```python
from build123d import *

# Parameters (mm, degrees)
RING_BASE_PROFILE_R        = 80.875
RING_BASE_PROFILE_R_2      = 70.375
RING_BASE_EXTRUSTION_DEPTH = 1.5
RING_LIP_PROFILE_W         = 0.8
RING_LIP_PROFILE_H         = 4
LED_CHANNEL_PROFILE_R      = 79.425
LED_CHANNEL_PROFILE_R_2    = 71.825
LED_CHANNEL_CUT_DEPTH      = 0.75


with BuildPart() as part:
    # Ring Base Profile → Ring Base Extrustion (new body)
    with BuildSketch(Plane(origin=(0, 0, 0), x_dir=(1, 0, 0), z_dir=(0, 1, 0))):
        with Locations(Location((0, 0, 0), (0, 0, 270))):
            Circle(RING_BASE_PROFILE_R)
        with Locations(Location((0, 0, 0), (0, 0, 270))):
            Circle(RING_BASE_PROFILE_R_2, mode=Mode.SUBTRACT)
    extrude(amount=RING_BASE_EXTRUSTION_DEPTH)

    # Ring Lip: sweep along a curve in space
    with BuildLine() as ring_lip_path:
        ThreePointArc((0, 1.5, 80.875), (57.187260928, 1.5, 57.187260928), (80.875, 1.5, 0))
        ThreePointArc((80.875, 1.5, 0), (57.187260928, 1.5, -57.187260928), (0, 1.5, -80.875))
        ThreePointArc((0, 1.5, -80.875), (-57.187260928, 1.5, -57.187260928), (-80.875, 1.5, 0))
        ThreePointArc((-80.875, 1.5, 0), (-57.187260928, 1.5, 57.187260928), (0, 1.5, 80.875))
    # Ring Lip Profile → Ring Lip (sweep)
    with BuildSketch(Plane.XY):
        with BuildLine():
            Line((-80.875, 1.5), (-80.875, -0.35))
            ThreePointArc((-80.875, -0.35), (-81.275, -0.75), (-80.875, -1.15))
            Line((-80.875, -1.15), (-80.875, -2.5))
            Line((-80.875, -2.5), (-81.675, -2.5))
            Line((-81.675, -2.5), (-81.675, 1.5))
            Line((-81.675, 1.5), (-80.875, 1.5))
        make_face()
        with Locations((-69.975, -0.5)):
            Rectangle(RING_LIP_PROFILE_W, RING_LIP_PROFILE_H)
    sweep(path=ring_lip_path.line)

    # LED Channel Profile → LED Channel Cut (cut)
    with BuildSketch(Plane.XZ):
        with Locations(Location((0, 0, 0), (0, 0, 270))):
            Circle(LED_CHANNEL_PROFILE_R)
        with Locations(Location((0, 0, 0), (0, 0, 270))):
            Circle(LED_CHANNEL_PROFILE_R_2, mode=Mode.SUBTRACT)
    extrude(amount=-LED_CHANNEL_CUT_DEPTH, mode=Mode.SUBTRACT)


solid = part.part
```
Design review of the part built by this model. Coordinates are the model's own, in mm. A direction names the side the tool comes from. Round coordinates to 2 decimals unless told otherwise and drop trailing zeros. Write each loop counter-clockwise with the first axis right and the second up, starting at its lowest first coordinate (ties: lowest second). Pieces come first, ordered by that corner, then holes. Notation, with made-up numbers: (71.5, 43.25) -> (107.5, 43.25) arc R19 cw to (107.5, 68.25) -> close; hole circle Ø9 at (65, 87.25). An arc over 180 degrees is marked (long way). Write item = value, one per line. Start each with the question number.
1) Mouldability with a two-part tool opening along Z and no side actions: class faces 3 (the face through (-53, 0, 48)), 4 (the face through (-59.4, -2.5, 36.9)) as +Z half, -Z half, draft (parallel to the pull), parting line (faces both ways), or undercut.
2) Clearance check with flat-ended pins moving along their axes: pin 1 (1.5 mm diameter, centred on x = -31.5, y = -1.5, fed in from -Z); pin 2 (2 mm diameter, centred on y = 0, z = -25, fed in from -X); pin 3 (1.5 mm diameter, centred on y = -1, z = -32, fed in from -X). State where each tip first meets the part, or that it passes through.
3) Wall thickness on probe 1 along Z at (x, y) = (24, -2.2); probe 2 along Z at (x, y) = (-27.5, -0.2); probe 3 along X at (y, z) = (-1.6, -34): over which ranges is each line inside the solid? List them lowest first. Write a range as from..to.
4) Tool access review of faces 1 (the face through (66.97, 0.37, -42.7)), 2 (the face through (68, 1.5, -17)): name each direction out of +Z, -Z, +X, -X, +Y, -Y from which nothing blocks a thin tool from reaching the whole face with its end or side.
5) Take a section at A-A, the plane y = -1.8. State the section outline as (x, z) points (3 decimals), plus the area to 3 significant figures.
Results list:
q1.face_3 = undercut
q1.face_4 = draft
q2.pin_1 = -75.67
q2.pin_2 = -78.07
q2.pin_3 = -75.46
q3.probe_1 = -78.07..-77.23, -66.16..-65.3, 65.3..66.16, 77.23..78.07
q3.probe_2 = -76.91..-76.06, -64.78..-63.91, 63.91..64.78, 76.06..76.91
q3.probe_3 = -74.26..-73.38, -61.62..-60.7, 60.7..61.62, 73.38..74.26
q4.face_1 = -Y
q4.face_2 = +Z, -Z, +X, -X, +Y
q5.outline = circle Ø163.35 at (0, 0); circle Ø140.75 at (0, 0); hole circle Ø161.75 at (0, 0); hole circle Ø139.15 at (0, 0)
q5.area = 760 mm²
